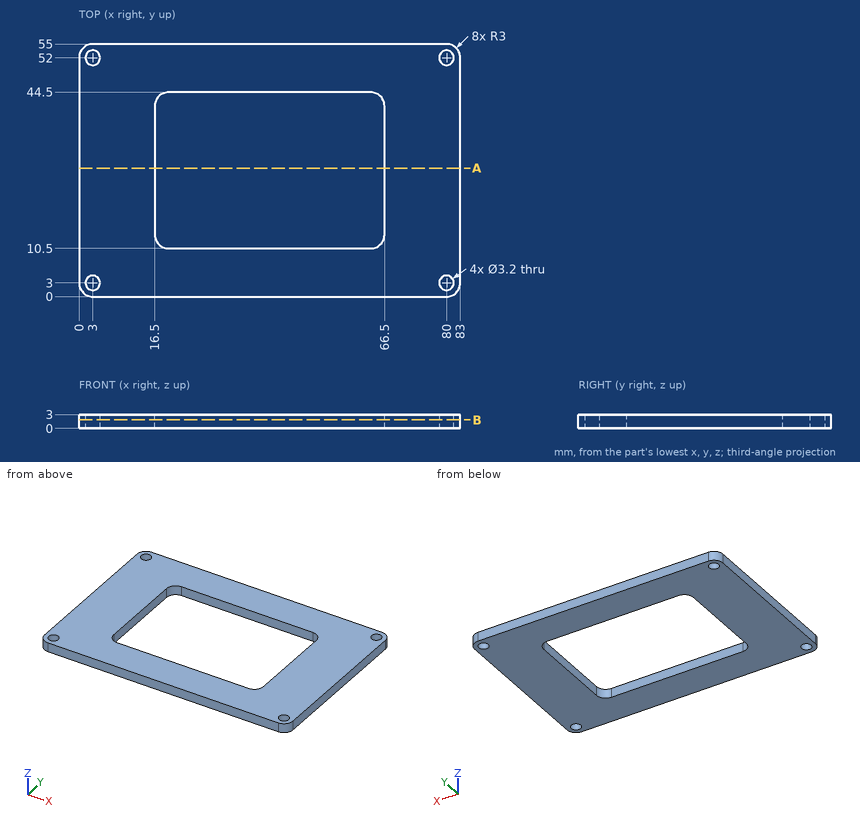
Source: three-view drawing plus pictorial views. Frame: mm from the lowest corner of the part. Give positions to 0.01 mm unless a question says otherwise; leave off trailing zeros. Write each loop counter-clockwise with the first axis right and the second up, starting at its lowest first coordinate (ties: lowest second). Pieces come first, ordered by that corner, then holes. Notation, with made-up numbers: (12.5, -2.75) -> (50.5, -2.75) arc R17 ccw to (50.5, 1.25) -> close; hole circle Ø11 at (46.5, 55). An arc over 180 degrees is marked (long way). Answer in a Markdown table with one row per item.
(1) Section query B-B on z = 1.85. Return loops of the section in (x, y), then the cut area to 3 significant figures.
Answers below:
| item | result |
|---|---|
| outline | (0, 3) arc R3 ccw to (3, 0) -> (80, 0) arc R3 ccw to (83, 3) -> (83, 52) arc R3 ccw to (80, 55) -> (3, 55) arc R3 ccw to (0, 52) -> close; hole circle Ø3.2 at (3, 3); hole circle Ø3.2 at (3, 52); hole (16.5, 13.5) arc R3 ccw to (19.5, 10.5) -> (63.5, 10.5) arc R3 ccw to (66.5, 13.5) -> (66.5, 41.5) arc R3 ccw to (63.5, 44.5) -> (19.5, 44.5) arc R3 ccw to (16.5, 41.5) -> close; hole circle Ø3.2 at (80, 3); hole circle Ø3.2 at (80, 52) |
| area | 2,830 mm^2 |
(2) Section query A-A on y = 28. Return loops of the section in (x, z), then the cut area to 3 significant figures.
Answers below:
| item | result |
|---|---|
| outline | (0, 0) -> (16.5, 0) -> (16.5, 3) -> (0, 3) -> close; (66.5, 0) -> (83, 0) -> (83, 3) -> (66.5, 3) -> close |
| area | 99.0 mm^2 |
(3) Ray query, line 1 along Y through (x, z) = (80, 2.2); line 2 along X through (y, z) = (41.5, 1.15); line 3 along Y through (x, z) = (62.5, 1.1). Return the intervals inside material, ascending. Write a range as [from, to].
Answers below:
| item | result |
|---|---|
| line 1 | [0, 1.4], [4.6, 50.4], [53.6, 55] |
| line 2 | [0, 16.5], [66.5, 83] |
| line 3 | [0, 10.5], [44.5, 55] |
